Model file for the job. Use its own axes, mm. A direction names the side the tool comes from. Coordinates: 2 decimals unless noted, no trailing zeros. Loops run counter-clockwise (first coordinate to the right, second up) from the corner with the lowest first, then second, coordinate; pieces in that order, holes last. Notation, with made-up numbers: M -25,-39 L 14,-39 A15 cw 14,-35 Z; hole C 49.5,22 d7. An arc over 180 degrees is marked long. One line per question, with ' | ' between items. Start each with the question number.
```python
from build123d import *

# Parameters (mm, degrees)
SUPPORTOMOTORE_DEPTH       = 30
SCHIZZO22_W                = 5
SCHIZZO22_H                = 3.93366559
ESTENSIONEBASEVITI_DEPTH   = 30
SCHIZZO12_W                = 41
SCHIZZO12_H                = 37
SUPPORTOESC_DEPTH          = 4
SCHIZZO13_W                = 7
SCHIZZO13_H                = 4
FORIFASCETTA_DEPTH         = 4
PILASTRINIESC_REACH        = 51.759
PILASTRINIESC_END_RADIUS   = 11
SCHIZZO14_R                = 3
SCHIZZO15_W                = 3
SCHIZZO15_H                = 30
BASEMOTORE_DEPTH           = 34
SCHIZZO16_R                = 1.5
SCHIZZO16_R_2              = 3.5
FORIMOTORE_DEPTH           = 3
CONTROVENTODESTRO_DEPTH    = 4
SUPPORTOBASEMOTORE_DEPTH   = 4
FORIVITIAGGANCI_REACH      = 59.738
SCHIZZO20_R                = 2
FORODADO_DEPTH             = 3
FOROTIRANTEANTERIORE_REACH = 63.131
SCHIZZO24_R                = 2.25


with BuildPart() as part:
    # Schizzo1 → SupportoMotore (new body)
    with BuildSketch(Plane.XY):
        with BuildLine():
            Line((-2.5, -10.712142643), (-2.5, -15.712142643))
            Line((-2.5, -15.712142643), (-7.5, -15.712142643))
            Line((-7.5, -15.712142643), (-7.5, -8.04673847))
            ThreePointArc((-7.5, -8.04673847), (-10.999946955, -0.034161219), (-7.549834435, 8))
            Line((-7.549834435, 8), (-15.935446939, 8))
            Line((-15.935446939, 8), (-15.935446939, 11))
            Line((-15.935446939, 11), (14.064553061, 11))
            Line((14.064553061, 11), (14.064553061, 8))
            Line((14.064553061, 8), (7.549834435, 8))
            ThreePointArc((7.549834435, 8), (10.999946955, -0.034161219), (7.5, -8.04673847))
            Line((7.5, -8.04673847), (7.5, -15.712142643))
            Line((7.5, -15.712142643), (2.5, -15.712142643))
            Line((2.5, -15.712142643), (2.5, -10.712142643))
            Line((2.5, -10.712142643), (2.5, -8.645808233))
            ThreePointArc((2.5, -8.645808233), (0, 9), (-2.5, -8.645808233))
            Line((-2.5, -8.645808233), (-2.5, -10.712142643))
        make_face()
    extrude(amount=SUPPORTOMOTORE_DEPTH)

    # Schizzo22 → EstensioneBaseViti (add)
    with BuildSketch(Plane(origin=(0, 0, 0), x_dir=(-1, 0, 0), z_dir=(0, 0, -1))):
        with Locations((-5, -17.678975438)):
            Rectangle(SCHIZZO22_W, SCHIZZO22_H)
        with Locations((5, -17.678975438)):
            Rectangle(SCHIZZO22_W, SCHIZZO22_H)
    extrude(amount=-ESTENSIONEBASEVITI_DEPTH)

    # Schizzo12 → SupportoESC (add)
    with BuildSketch(Plane.ZY.offset(15.935446939)):
        with Locations((9.5, -7.5)):
            Rectangle(SCHIZZO12_W, SCHIZZO12_H)
    extrude(amount=SUPPORTOESC_DEPTH)

    # Schizzo13 → ForiFascetta (cut)
    with BuildSketch(Plane.ZY.offset(19.935446939)):
        with Locations((-2.5, 6)):
            Rectangle(SCHIZZO13_W, SCHIZZO13_H)
        with Locations((21.5, 6)):
            Rectangle(SCHIZZO13_W, SCHIZZO13_H)
        with Locations((21.5, -21)):
            Rectangle(SCHIZZO13_W, SCHIZZO13_H)
        with Locations((-2.5, -21)):
            Rectangle(SCHIZZO13_W, SCHIZZO13_H)
    extrude(amount=-FORIFASCETTA_DEPTH, mode=Mode.SUBTRACT)

    # PilastriniESC: up to this cylinder (the profile starts outside it)
    pilastriniesc_end = Plane(origin=(0, 0, 15), z_dir=(0, 0, -1)) * Cylinder(PILASTRINIESC_END_RADIUS, 140.518, mode=Mode.PRIVATE)
    # Schizzo14 → PilastriniESC (add, up to the surface)
    with BuildSketch(Plane(origin=(-15.935446939, 0, 0), x_dir=(0, 0, -1), z_dir=(1, 0, 0)), mode=Mode.PRIVATE) as pilastriniesc_sk1:
        with Locations(Location((-8, -3.5, 0), (0, 0, 270))):
            Circle(SCHIZZO14_R)
    pilastriniesc_tool1 = extrude(pilastriniesc_sk1.sketch, amount=PILASTRINIESC_REACH, mode=Mode.PRIVATE) - pilastriniesc_end
    add(pilastriniesc_tool1.solids().sort_by_distance((-15.935447, -3.5, 8))[0])
    # Schizzo14 → PilastriniESC (add, up to the surface)
    with BuildSketch(Plane(origin=(-15.935446939, 0, 0), x_dir=(0, 0, -1), z_dir=(1, 0, 0)), mode=Mode.PRIVATE) as pilastriniesc_sk2:
        with Locations(Location((-22, -3.5, 0), (0, 0, 270))):
            Circle(SCHIZZO14_R)
    pilastriniesc_tool2 = extrude(pilastriniesc_sk2.sketch, amount=PILASTRINIESC_REACH, mode=Mode.PRIVATE) - pilastriniesc_end
    add(pilastriniesc_tool2.solids().sort_by_distance((-15.935447, -3.5, 22))[0])

    # Schizzo15 → BaseMotore (add)
    with BuildSketch(Plane.ZY.offset(19.935446939)):
        with Locations((18.5, 26)):
            Rectangle(SCHIZZO15_W, SCHIZZO15_H)
    extrude(amount=-BASEMOTORE_DEPTH)

    # Schizzo16 → ForiMotore (cut)
    with BuildSketch(Plane.XY.offset(20)):
        with Locations((-8.592301188, 31.656854249)):
            Circle(SCHIZZO16_R)
        with Locations((2.721407311, 31.656854249)):
            Circle(SCHIZZO16_R)
        with Locations((2.721407311, 20.343145751)):
            Circle(SCHIZZO16_R)
        with Locations((-8.592301188, 20.343145751)):
            Circle(SCHIZZO16_R)
        with Locations((-2.935446939, 26)):
            Circle(SCHIZZO16_R_2)
    extrude(amount=-FORIMOTORE_DEPTH, mode=Mode.SUBTRACT)

    # Schizzo17 → ControventoDestro (add)
    with BuildSketch(Plane.ZY.offset(19.935446939)):
        Polygon((17, 41), (0, 11), (17, 11), align=None)
        Polygon((15, 15), (15, 21), (9.675284069, 24.017339028), (7.101692816, 19.475707404), align=None, mode=Mode.SUBTRACT)
        Polygon((15, 33.413896553), (10.53314782, 25.531216235), (15, 23), align=None, mode=Mode.SUBTRACT)
        Polygon((3.432125287, 13), (15, 13), (6.243829065, 17.961830197), align=None, mode=Mode.SUBTRACT)
    controventodestro = extrude(amount=-CONTROVENTODESTRO_DEPTH)

    # ControventoSinistro: ControventoDestro across plane
    add(controventodestro.mirror(Plane(origin=(-2.935446939, 0, 0), x_dir=(0, 0, 1), z_dir=(1, 0, 0))))

    # Schizzo19 → SupportoBaseMotore (add)
    with BuildSketch(Plane.XY.offset(20)):
        with BuildLine():
            Line((-19.935446939, 11), (14.064553061, 11))
            Line((14.064553061, 11), (14.064553061, 17))
            Line((14.064553061, 17), (8.624072947, 17))
            ThreePointArc((8.624072947, 17), (-2.935446939, 11.35), (-14.494966825, 17))
            Line((-14.494966825, 17), (-19.935446939, 17))
            Line((-19.935446939, 17), (-19.935446939, 11))
        make_face()
    extrude(amount=SUPPORTOBASEMOTORE_DEPTH)

    # ForiVitiAgganci: up to this face of the body (flat: up to its plane)
    forivitiagganci_end = Plane(part.part.faces().sort_by_distance((-7.5, -13.846273351, 15))[0])
    # Schizzo20 → ForiVitiAgganci (cut, up to the picked face)
    with BuildSketch(Plane(origin=(7.5, 0, 0), x_dir=(0, 0, -1), z_dir=(1, 0, 0)), mode=Mode.PRIVATE) as forivitiagganci_sk1:
        with Locations((-20, -13.846273351)):
            Circle(SCHIZZO20_R)
    forivitiagganci_tool1 = split(extrude(forivitiagganci_sk1.sketch, amount=-FORIVITIAGGANCI_REACH, mode=Mode.PRIVATE), bisect_by=forivitiagganci_end, keep=Keep.BOTH, mode=Mode.PRIVATE)
    # Schizzo20 → ForiVitiAgganci (cut, up to the picked face)
    with BuildSketch(Plane(origin=(7.5, 0, 0), x_dir=(0, 0, -1), z_dir=(1, 0, 0)), mode=Mode.PRIVATE) as forivitiagganci_sk2:
        with Locations((-10, -13.846273351)):
            Circle(SCHIZZO20_R)
    forivitiagganci_tool2 = split(extrude(forivitiagganci_sk2.sketch, amount=-FORIVITIAGGANCI_REACH, mode=Mode.PRIVATE), bisect_by=forivitiagganci_end, keep=Keep.BOTH, mode=Mode.PRIVATE)
    add(forivitiagganci_tool1.solids().sort_by(Axis((7.5, -13.846273, 20), (-1, 0, 0)))[0], mode=Mode.SUBTRACT)
    add(forivitiagganci_tool2.solids().sort_by(Axis((7.5, -13.846273, 10), (-1, 0, 0)))[0], mode=Mode.SUBTRACT)

    # Schizzo21 → SvasaturaViteDestra (revolve, cut)
    with BuildSketch(Plane.XY.offset(10), mode=Mode.PRIVATE) as svasaturavitedestra_sk:
        Polygon((7.5, -9.846273351), (4.5, -11.846273351), (4.5, -13.846273351), (7.5, -13.846273351), align=None)
    svasaturavitedestra = revolve(svasaturavitedestra_sk.sketch.rotate(Axis((4.5, -13.846273351, 10), (1, 0, 0)), 270), axis=Axis((4.5, -13.846273351, 10), (1, 0, 0)), mode=Mode.SUBTRACT)

    # SvasaturaViteSinistra: SvasaturaViteDestra across plane
    add(svasaturavitedestra.mirror(Plane.XY.offset(15)), mode=Mode.SUBTRACT)

    # Schizzo23 → ForoDado (cut)
    with BuildSketch(Plane.ZY.offset(7.5)):
        Polygon((6.102885683, -11.596273351), (6.102885683, -16.096273351), (10, -18.346273351), (13.897114317, -16.096273351), (13.897114317, -11.596273351), (10, -9.346273351), align=None)
        Polygon((16.102885683, -11.596273351), (16.102885683, -16.096273351), (20, -18.346273351), (23.897114317, -16.096273351), (23.897114317, -11.596273351), (20, -9.346273351), align=None)
    extrude(amount=-FORODADO_DEPTH, mode=Mode.SUBTRACT)

    # Schizzo24 → ForoTiranteAnteriore (cut, up to next)
    with BuildSketch(Plane.ZY.offset(19.935446939), mode=Mode.PRIVATE) as forotiranteanteriore_sk1:
        with Locations(Location((9.5, -21, 0), (0, 0, 270))):
            Circle(SCHIZZO24_R)
    forotiranteanteriore_tool1 = extrude(forotiranteanteriore_sk1.sketch, amount=-FOROTIRANTEANTERIORE_REACH, mode=Mode.PRIVATE) & part.part
    add(forotiranteanteriore_tool1.solids().sort_by_distance((-19.935447, -21, 9.5))[0], mode=Mode.SUBTRACT)


solid = part.part
```
(1) Drill centre lines: line 1 (X direction, y = -0.5, z = 15); line 2 (X direction, y = -12, z = 5); line 3 (Z direction, x = -18, y = -21). Where is each one in solid material? Low to high. Write a range as [from, to].
(2) Pin check, flat tips, straight feed: P1, Ø3.5, axis at x = 2.72, y = 31.66, coming from the -Z side; P2, Ø3, axis at x = 10, y = 1.5, coming from the -Z side; P3, Ø10, axis at y = 21, z = 20.5, coming from the -X side; P4, Ø1.5, axis at x = 4, z = 25, coming from the +Y side. Stop position of each tip, or through.
(3) Band-saw the part on B-B on y = -21. Write the cut outline in (x, z).
(4) Band-saw the part on C-C on x = -1.5. Write the cut outline in (y, z), then the cut area to 3 significant figures.
(5) 3-axis set-ups, long thin cutter, end or side, ignore diameter. For faces 1 (the face through (-3, 11, 27)), 2 (the face through (-17.96, 15.45, 10.68)), 3 (the face through (10.065, 23, 12)), 4 (the face through (-6, -10.5, 12)): which of +Z, -Z, +X, -X, +Y, -Y reach the whole face in a straight line?
(6) Band-saw the part on A-A on z = -4. Write the cut outline in (x, y).
(7) Band-saw the part on D-D on z = 27.5. Write the cut outline in (x, y), then the cut area to 3 significant figures.
(8) Two-plate mould, pull along Y, no slides. Class faces 5 (the face through (-18, -19, 21)), 6 (the face through (-17.96, 29.53, 12.8)), 7 (the face through (-17, 17, 22)), 8 (the face through (-18, -26, 9)): pulls with the +Y half, pulls with the -Y half, needs draft (parallel to the pull), parting line crosses it, or undercut.
Computed values:
1) line 1: [-19.94, -15.94], [-10.99, -8.99], [8.99, 10.99] | line 2: [-19.94, -15.94], [-7.5, -2.5], [2.5, 7.5] | line 3: [-11, -6], [1, 7.25], [11.75, 18], [25, 30]
2) P1: z = 17 | P2: z = 0 | P3: x = -19.94 | P4: y = 11
3) outline: M -19.94,-11 L -15.94,-11 L -15.94,-6 L -19.94,-6 Z; M -19.94,1 L -15.94,1 L -15.94,7.25 L -19.94,7.25 Z; M -19.94,11.75 L -15.94,11.75 L -15.94,18 L -19.94,18 Z; M -19.94,25 L -15.94,25 L -15.94,30 L -19.94,30 Z
4) outline: M 8.87,0 L 11,0 L 11,17 L 22.81,17 L 22.81,20 L 11.42,20 L 11.42,24 L 11,24 L 11,30 L 8.87,30 Z; M 29.19,17 L 41,17 L 41,20 L 29.19,20 Z | area: 136 mm^2
5) face 1: +Z, +X, -X, +Y | face 2: +X, -X | face 3: -Z, +Y | face 4: none
6) outline: M -19.94,-26 L -15.94,-26 L -15.94,-23 L -19.94,-23 Z; M -19.94,-19 L -15.94,-19 L -15.94,4 L -19.94,4 Z; M -19.94,8 L -15.94,8 L -15.94,11 L -19.94,11 Z
7) outline: M -19.94,-26 L -15.94,-26 L -15.94,8 L -7.55,8 A11 ccw -7.5,-8.05 L -7.5,-19.65 L -2.5,-19.65 L -2.5,-8.65 A9 cw long 2.5,-8.65 L 2.5,-19.65 L 7.5,-19.65 L 7.5,-8.05 A11 ccw 7.55,8 L 14.06,8 L 14.06,11 L -19.94,11 Z | area: 422 mm^2
8) face 5: undercut | face 6: undercut | face 7: pulls with the +Y half | face 8: pulls with the -Y half
